```python
from build123d import *

# Parameters (mm, degrees)
F1_DEPTH      = 12.7
F2_R          = 15.875
F2_R_2        = 9.525
F3_DEPTH      = 6.35
F3_DEPTH_BACK = 19.05
F4_R          = 9.525
F5_DEPTH      = 25.4
F7_DEPTH      = 25.401
F8_R          = 4.7625
F8_R_2        = 3.81
F8_R_3        = 3.175
F8_R_4        = 4.2961277226
F9_DEPTH      = 19.051
F12_DEPTH     = 19.051
F14_DEPTH     = 25.4


# Not quite as in the source:
# - after a boolean that leaves OpenCascade's solid faulty, fix() repairs it


with BuildPart() as f1:
    # F0 (on Front) → F1 (new body)
    with BuildSketch(Plane.XZ):
        with BuildLine():
            ThreePointArc((-12.1609555345, 5.6707466962), (-6.7090649051, 1.4873638808), (0, 0))
            Line((0, 0), (79.375, 0))
            ThreePointArc((79.375, 0), (95.885, 16.51), (79.375, 33.02))
            Line((79.375, 33.02), (9.525, 33.02))
            ThreePointArc((9.525, 33.02), (7.3531720899, 33.402951858), (5.4432986785, 34.5056177862))
            Line((5.4432986785, 34.5056177862), (-30.3843620081, 64.5685946542))
            ThreePointArc((-30.3843620081, 64.5685946542), (-46.6383026366, 63.8589322804), (-47.3479650105, 47.6049916518))
            Line((-47.3479650105, 47.6049916518), (-12.1609555345, 5.6707466962))
        make_face()
    extrude(amount=F1_DEPTH)

    # F2 (on face) → F3 (join, two sides)
    with BuildSketch(Plane.XZ.offset(12.7)) as f3_sk:
        with Locations((0, 15.875)):
            Circle(F2_R)
        with Locations((0, 15.875)):
            Circle(F2_R_2, mode=Mode.SUBTRACT)
    extrude(amount=F3_DEPTH)
    extrude(f3_sk.sketch, amount=-F3_DEPTH_BACK)

    add(f1.part.fix(), mode=Mode.REPLACE)

    # F4 (on face) → F5 (cut)
    with BuildSketch(Plane.XZ.offset(12.7)):
        with Locations((0, 15.875)):
            Circle(F4_R)
    extrude(amount=-F5_DEPTH, mode=Mode.SUBTRACT)

    # F6 (on face) → F7 (cut, through all)
    with BuildSketch(Plane.XZ.offset(19.05)):
        with BuildLine():
            Line((-8.3178005381, 11.2338989228), (-11.2676186575, 8.2840808033))
            Line((-11.2676186575, 8.2840808033), (-8.034726454, 5.0511885997))
            Line((-8.034726454, 5.0511885997), (-5.1946960102, 7.8912190435))
            ThreePointArc((-5.1946960102, 7.8912190435), (-6.959904305, 9.3722807946), (-8.3178005381, 11.2338989228))
        make_face()
    extrude(amount=-F7_DEPTH, mode=Mode.SUBTRACT)

    # F8 (on face) → F9 (cut, through all)
    with BuildSketch(Plane.XZ.offset(12.7)):
        with Locations((78.74, 16.51)):
            Circle(F8_R)
        with Locations((41.91, 23.495)):
            Circle(F8_R_2)
        with Locations((41.91, 9.525)):
            Circle(F8_R_2)
        with Locations((-24.765, 38.735)):
            Circle(F8_R_3)
        with Locations((-38.6896171983, 57.7962485902)):
            Circle(F8_R_4)
    extrude(amount=-F9_DEPTH, mode=Mode.SUBTRACT)

    # F11 (on face) → F12 (cut, through all)
    with BuildSketch(Plane.XZ.offset(12.7)):
        with BuildLine():
            Line((95.758, 18.5538715713), (95.758, 14.4661284287))
            ThreePointArc((95.758, 14.4661284287), (95.885, 16.51), (95.758, 18.5538715713))
        make_face()
        with BuildLine():
            ThreePointArc((95.758, 18.5538715713), (95.885, 16.51), (95.758, 14.4661284287))
            Line((95.758, 14.4661284287), (95.758, 13.97))
            Line((95.758, 13.97), (97.3146509769, 13.97))
            Line((97.3146509769, 13.97), (97.3146509769, 19.05))
            Line((97.3146509769, 19.05), (95.758, 19.05))
            Line((95.758, 19.05), (95.758, 18.5538715713))
        make_face()
    extrude(amount=-F12_DEPTH, mode=Mode.SUBTRACT)

    # F13 (on face) → F14 (join)
    with BuildSketch(Plane.XZ.offset(19.05)):
        with BuildLine():
            Line((5.9313747803, 23.3278127721), (7.0446438565, 22.2858203792))
            ThreePointArc((7.0446438565, 22.2858203792), (6.5088940652, 22.8291299274), (5.9313747803, 23.3278127721))
        make_face()
    extrude(amount=-F14_DEPTH)


solid = f1.part
```
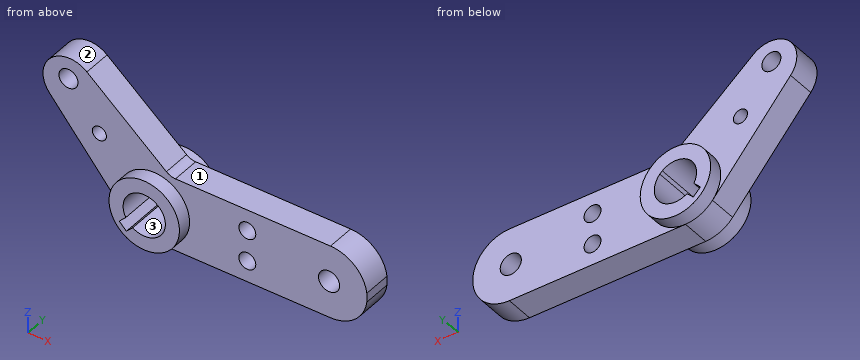
Verification items for the finished model (mm, model axes). Face numbers are marked on the shaded views. Give positions to 0.01 mm unless a question says otherwise; leave off trailing zeros. Order: outer loops, then holes, each group sorted by start corner. A loop starts at its lowest first (then second) coordinate and runs counter-clockwise, first axis right, second up. Notation, with made-up numbers: M 21,41.5 L 42,41.5 A24 cw 42,59.5 Z; hole C -27,14.25 d10. An arc over 180 degrees is marked long. Answer in a Markdown table with one row per item. Add a question column.
Item 1: Mould release check, pull along Z, two halves, no side actions. Record for the marked faces 1, 2 and 3: released by +Z, released by -Z, zero draft, split by the parting line, or undercut.
Item 2: Section check D-D, the plane x = 60.5. Enter the section's corners in (y, z), and give its area (3 significant figures).
Item 3: Section check A-A, the plane x = 41.91. Enter the section's corners in (y, z) (3 decimals).
Item 4: Section check C-C, the plane y = -9.75. State how many separate pieces and enclosed holes the cut face has, and give its area (3 significant figures).
Item 5: Section check B-B, the plane y = -15.5. Enter the section's corners in (x, z) (3 decimals), and give its area (3 significant figures).
Item 6: Gauge pin test, flat ends, axial feed: pin 1 (6 mm diameter, centred on x = 41.91, z = 23.495, fed in from +Y); pin 2 (6 mm diameter, centred on y = -10.5, z = 28.5, fed in from -X); pin 3 (15 mm diameter, centred on x = 78.74, z = 16.51, fed in from -Y); pin 4 (8 mm diameter, centred on x = 11.5, y = -12, fed in from +Z). Record the tip position at first contact, or that the pin passes through.
Item 7: Scan lines: probe 1 along Z at (x, y) = (78.74, -5.75); probe 2 along Z at (x, y) = (49.5, -6); probe 3 along Y at (x, z) = (74, 23). Record each from-to range of solid material in increasing order. Write a range as from..to.
Filled sheet:
| question | item | result |
|---|---|---|
| 1 | face 1 | released by +Z |
| 1 | face 2 | split by the parting line |
| 1 | face 3 | undercut |
| 2 | outline | M -12.7,0 L 0,0 L 0,33.02 L -12.7,33.02 Z |
| 2 | area | 419 mm^2 |
| 3 | outline | M -12.7,0 L 0,0 L 0,5.715 L -12.7,5.715 Z; M -12.7,13.335 L 0,13.335 L 0,19.685 L -12.7,19.685 Z; M -12.7,27.305 L 0,27.305 L 0,33.02 L -12.7,33.02 Z |
| 4 | separate pieces | 1 |
| 4 | enclosed holes | 6 |
| 4 | area | 4,290 mm^2 |
| 5 | outline | C 0,15.875 d31.75; hole M -11.268,8.284 L -8.035,5.051 L -5.195,7.891 A9.525 ccw 7.045,22.286 L 5.931,23.328 A9.525 ccw -8.318,11.234 Z |
| 5 | area | 489 mm^2 |
| 6 | pin 1 | passes through |
| 6 | pin 2 | stops at x = -33.83 |
| 6 | pin 3 | stops at y = -12.7 |
| 6 | pin 4 | stops at z = 33.35 |
| 7 | probe 1 | z = 0..11.75, 21.27..33.02 |
| 7 | probe 2 | z = 0..33.02 |
| 7 | probe 3 | y = -12.7..0 |
